from build123d import *

# Parameters (mm, degrees)
SKETCH_2_W               = 1.5
SKETCH_2_H               = 1.2
CUT_EXTRUDE_1_DEPTH      = 6
CUT_EXTRUDE_1_DEPTH_BACK = 6
CHAMFER_1_SIZE           = 0.6
FILLET_1_R               = 1
FILLET_2_R               = 0.4


with BuildPart() as part:
    # Эскиз1 → Повернуть1 (revolve)
    with BuildSketch(Plane(origin=(0, 0, 0), x_dir=(1, 0, 0), z_dir=(0, 1, 0))):
        Polygon((0, 0), (-5, 0), (-5, 3), (-2.5, 3), (-2.5, 23), (0, 23), align=None)
    revolve(axis=Axis((0, 0, -23), (0, 0, 1)))

    # Эскиз2 → Вырез-Вытянуть1 (cut, two sides)
    with BuildSketch(Plane(origin=(0, 0, 0), x_dir=(0, 0, -1), z_dir=(1, 0, 0))) as cut_extrude_1_sk:
        with Locations((0.75, 0)):
            Rectangle(SKETCH_2_W, SKETCH_2_H)
    extrude(amount=CUT_EXTRUDE_1_DEPTH, mode=Mode.SUBTRACT)
    extrude(cut_extrude_1_sk.sketch, amount=-CUT_EXTRUDE_1_DEPTH_BACK, mode=Mode.SUBTRACT)

    # Фаска1
    chamfer_1_edges = [part.edges().sort_by_distance(p)[0] for p in [
        (2.5, 0, -23),
    ]]
    chamfer(chamfer_1_edges, length=CHAMFER_1_SIZE)

    # Скругление1
    fillet_1_edges = [part.edges().sort_by_distance(p)[0] for p in [
        (0, 5, 0),
        (0, -5, 0),
    ]]
    fillet(fillet_1_edges, radius=FILLET_1_R)

    # Скругление2
    fillet_2_edges = [part.edges().sort_by_distance(p)[0] for p in [
        (2.5, 0, -3),
    ]]
    fillet(fillet_2_edges, radius=FILLET_2_R)


solid = part.part
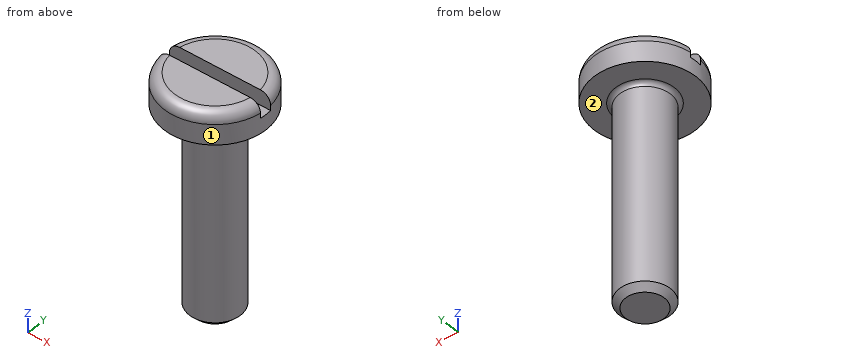
Input: part model. Units: mm. Frame: model coordinates. Face numbers are marked on the shaded views. A direction names the side the tool comes from. Coordinates: 2 decimals unless noted, no trailing zeros. Loops run counter-clockwise (first coordinate to the right, second up) from the corner with the lowest first, then second, coordinate; pieces in that order, holes last.
Q1. Cut plane C-C (z = -20.5). Output: boundary loops of the cut face in (x, y), then the cut area to 3 significant figures.
Q2. Cut plane B-B (x = 0). Output: boundary loops of the cut face in (y, z), then the cut area to 3 significant figures.
Q3. Set-up query: the marked faces 1 and 2. Return all of +Z, -Z, +X, -X, +Y, -Y with unobstructed straight access to the full face (end or side cutting, diameter ignored); none if empty.
Q4. Cut plane D-D (z = -2.25). Output: boundary loops of the cut face in (x, y).
Q5. Material intervals for line 1 (Z direction, x = 1.5, y = 0); line 2 (Z direction, x = -3.75, y = 1); line 3 (X direction, y = 0.25, z = -5), sorted ascending.
Q6. Cut plane A-A (y = 0). Output: boundary loops of the cut face in (x, z).
Q7. Contact query for flat-ended pins moving along their axis: pin 1 (3 mm diameter, centred on y = 0, z = -6, fed in from -X); pin 2 (1 mm diameter, centred on x = -0.5, z = -11, fed in from -Y); pin 3 (1.7 mm diameter, centred on x = -2, z = -0.5, fed in from +Y); pin 4 (3 mm diameter, centred on x = 2, y = 1, fed in from -Z). Output: stop coordinate, or through.
Working result:
1. outline: circle Ø5 at (0, 0)
1. area: 19.6 mm2
2. outline: (-5, -3) - (-2.9, -3) arc R0.4 cw to (-2.5, -3.4) - (-2.5, -22.4) - (-1.9, -23) - (1.9, -23) - (2.5, -22.4) - (2.5, -3.4) arc R0.4 cw to (2.9, -3) - (5, -3) - (5, -1) arc R1 ccw to (4, 0) - (0.6, 0) - (0.6, -1.5) - (-0.6, -1.5) - (-0.6, 0) - (-4, 0) arc R1 ccw to (-5, -1) - close
2. area: 127 mm2
3. face 1: +Z, -Z
3. face 2: -Z
4. outline: circle Ø10 at (0, 0)
5. line 1: z = -23 to -1.5
5. line 2: z = -3 to 0
5. line 3: x = -2.49 to 2.49
6. outline: (-5, -3) - (-2.9, -3) arc R0.4 cw to (-2.5, -3.4) - (-2.5, -22.4) - (-1.9, -23) - (1.9, -23) - (2.5, -22.4) - (2.5, -3.4) arc R0.4 cw to (2.9, -3) - (5, -3) - (5, -1.5) - (-5, -1.5) - close
7. pin 1: stops at x = -2.5
7. pin 2: stops at y = -2.5
7. pin 3: stops at y = 4.84
7. pin 4: stops at z = -23
